CAD build for the part. Positions are in the model's coordinates, mm. Round coordinates to 2 decimals unless told otherwise and drop trailing zeros. Loops run counter-clockwise (first coordinate to the right, second up) from the corner with the lowest first, then second, coordinate; pieces in that order, holes last.
from build123d import *

# Parameters (mm, degrees)
F1_DEPTH = 15
F3_D     = 5
F2_R     = 3
F4_DEPTH = 25


with BuildPart() as f1:
    # F0 (on Front) → F1 (new body)
    with BuildSketch(Plane.XZ):
        Polygon((-43.1142237037, 16.1099138111), (-43.1142237037, 6.1099138111), (56.8857762963, 6.1099138111), (56.8857762963, 26.1099138111), (-23.1142237037, 26.1099138111), align=None)
    extrude(amount=F1_DEPTH)

    # F3 (through all)
    with Locations(Plane.XY.offset(26.1099138111)):
        with Locations((1.8857762963, -7.5)):
            Hole(F3_D / 2)

    # F2 (on face) → F4 (cut)
    with BuildSketch(Plane.XY.offset(26.1099138111)):
        with Locations((46.8857762963, -7.5)):
            Circle(F2_R)
    extrude(amount=-F4_DEPTH, mode=Mode.SUBTRACT)


solid = f1.part
Item 1: Cut at C-C (y = -12.25). List the corners of the cut face in (x, z), plus the area to 3 significant figures.
Verdict:
outline: (-43.11, 6.11) - (56.89, 6.11) - (56.89, 26.11) - (-23.11, 26.11) - (-43.11, 16.11) - close
area: 1,900 mm2
Item 2: Cut at D-D (x = -24.5). List the corners of the cut face in (y, z).
Verdict:
outline: (-15, 6.11) - (0, 6.11) - (0, 25.42) - (-15, 25.42) - close
Item 3: Wall check: L1, parallel to X at y = -9, z = 9.5; L2, parallel to X at y = -4.75, z = 18.75; L3, parallel to Z at x = -38, y = -3.5. Give the ranges that are in metal, low to high.
Verdict:
L1: x = -43.11 to -0.11, 3.89 to 44.29, 49.48 to 56.89
L2: x = -37.83 to 45.69, 48.08 to 56.89
L3: z = 6.11 to 18.67
Item 4: Mould opens along X. For faces 1 (the cylindrical face through (49.747, -6.599, 16.25)), 2 (the flat face through (-32.97, -7.4, 21.18)), 3 (the flat face through (6, -7, 6.11)) say: released by +X, released by -X, zero draft, split by the parting line, or undercut.
Verdict:
face 1: undercut
face 2: released by -X
face 3: zero draft
Item 5: Cut at A-A (y = -7.5). List the corners of the cut face in (x, z), plus the area to 3 significant figures.
Verdict:
outline: (-43.11, 6.11) - (-0.61, 6.11) - (-0.61, 26.11) - (-23.11, 26.11) - (-43.11, 16.11) - close; (4.39, 6.11) - (43.89, 6.11) - (43.89, 26.11) - (4.39, 26.11) - close; (49.89, 6.11) - (56.89, 6.11) - (56.89, 26.11) - (49.89, 26.11) - close
area: 1,680 mm2
Item 6: Cut at B-B (z = 22.75). List the corners of the cut face in (x, y).
Verdict:
outline: (-29.83, -15) - (56.89, -15) - (56.89, 0) - (-29.83, 0) - close; hole circle Ø5 at (1.89, -7.5); hole circle Ø6 at (46.89, -7.5)
Item 7: Flat gauge pins, fed straight in: P1, Ø2, axis at y = -5, z = 18.5, coming from the -X side; P2, Ø3.5, axis at x = 46.89, y = -7.5, coming from the +Z side. Where does each tip first touch, or does it go through?
Verdict:
P1: stops at x = -40.33
P2: passes through
